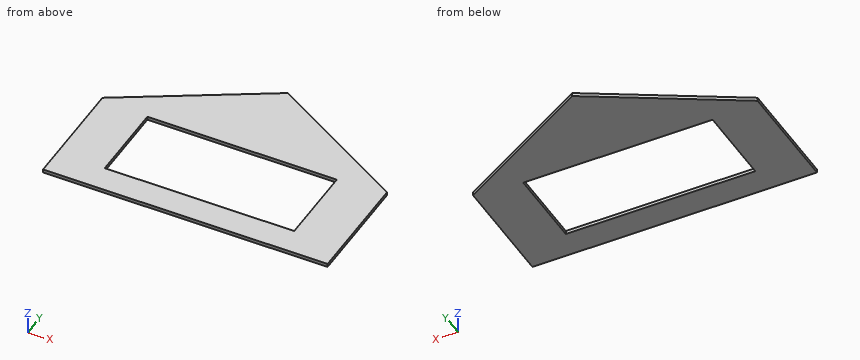
Autodesk Inventor part; units mm, degrees
ref_plane "YZ Plane" through (0, 0, 0) normal (1, 0, 0) x (0, 1, 0)
ref_plane "XZ Plane" through (0, 0, 0) normal (0, 1, 0) x (-1, 0, 0)
ref_plane "XY Plane" through (0, 0, 0) normal (0, 0, 1) x (1, 0, 0)
sketch "Sketch1" plane through (0, 0, 0) normal (0, 0, 1) x (1, 0, 0)
  line L0 (0, 0) -> (525.78, 0)
  line L1 (525.78, 0) -> (525.78, 209.2917)
  line L2 (525.78, 209.2917) -> (0, 209.2917)
  line L3 (0, 209.2917) -> (0, 0)
  line L4 (0, 209.2917) -> (262.89, 361.0713)
  line L5 (262.89, 361.0713) -> (525.78, 209.2917)
  point P0 (262.89, 209.2917)
  dimension "d0" = 525.78
  dimension "d1" = 209.2917
  dimension "d2" = 30
extrude "Extrusion1" add sketch "Sketch1" along normal blind 6.35
sketch "Sketch5" plane through (0, 0, 6.35) normal (0, 0, 1) x (1, 0, 0)
  line L0 (87.89, 50) -> (437.89, 50)
  line L1 (437.89, 50) -> (437.89, 200)
  line L2 (437.89, 200) -> (87.89, 200)
  line L3 (87.89, 200) -> (87.89, 50)
  line L4 (0, 0) -> (525.78, 0)
  point P0 (262.89, 200)
  point P1 (262.89, 361.0713)
  dimension "d16" = 350
  dimension "d17" = 150
  dimension "d21" = 50
extrude "Extrusion5" cut sketch "Sketch5" against normal through all
properties part number "BA10" material "ABS Plastic"
Can you work these out from the model? Positions are in its coordinate system, mm. Give positions to 0.01 mm unless a question says otherwise; leave off trailing zeros. Write each loop counter-clockwise with the first axis right and the second up, starting at its lowest first coordinate (ties: lowest second). Pieces come first, ordered by that corner, then holes. Notation, with made-up numbers: (24, 14.5) - (57, 14.5) arc R29 cw to (57, 50.5) - close; hole circle Ø9 at (72.25, -30.5). An arc over 180 degrees is marked (long way). Write item = value, one per line. Start each with the question number.
1. Please list where these lines run through material, in increasing order: line 1 (X direction, y = 193, z = 5.25); line 2 (Y direction, x = 419, z = 0.5); line 3 (Y direction, x = 132, z = 5.5).
2. Imagine slicing it at D-D (y = 273). Please give me the cut outline in (x, z), and give its area (3 significant figures).
3. Imagine slicing it at A-A (y = 170). Please give me the cut outline in (x, z), and give its area (3 significant figures).
4. Imagine slicing it at C-C (x = 319). Please give me the cut outline in (y, z).
5. Imagine slicing it at B-B (z = 3.25). Please give me the cut outline in (x, y), and give its area (3 significant figures).
6. For pin 1 (1.5 mm diameter, centred on x = 130.5, z = 5.5, fed in from +Y); pin 2 (2 mm diameter, centred on y = 273, z = 5.5, fed in from -X); pin 3 (3 mm diameter, centred on x = 202, z = 2.5, fed in from +Y), each with a flat end and sliding along its axis, tell me the tip position at first contact or that it passes through.
Worked answers:
q1.line_1 = 0 to 87.89, 437.89 to 525.78
q1.line_2 = 0 to 50, 200 to 270.94
q1.line_3 = 0 to 50, 200 to 285.5
q2.outline = (110.35, 0) - (415.43, 0) - (415.43, 6.35) - (110.35, 6.35) - close
q2.area = 1,940 mm2
q3.outline = (0, 0) - (87.89, 0) - (87.89, 6.35) - (0, 6.35) - close; (437.89, 0) - (525.78, 0) - (525.78, 6.35) - (437.89, 6.35) - close
q3.area = 1,120 mm2
q4.outline = (0, 0) - (50, 0) - (50, 6.35) - (0, 6.35) - close; (200, 0) - (328.68, 0) - (328.68, 6.35) - (200, 6.35) - close
q5.outline = (0, 0) - (525.78, 0) - (525.78, 209.29) - (262.89, 361.07) - (0, 209.29) - close; hole (87.89, 50) - (437.89, 50) - (437.89, 200) - (87.89, 200) - close
q5.area = 97,400 mm2
q6.pin_1 = 285.07
q6.pin_2 = 108.61
q6.pin_3 = 326.78
